from build123d import *

# Parameters (mm, degrees)
SKETCH1_R           = 63.5
BOSS_EXTRUDE1_DEPTH = 6.35
SKETCH2_R           = 20.6375
CUT_EXTRUDE1_DEPTH  = 91.02678768
SKETCH3_R           = 3.175
CUT_EXTRUDE2_DEPTH  = 91.02678768
SKETCH4_R           = 3.25
CUT_EXTRUDE3_DEPTH  = 91.02678768


with BuildPart() as part:
    # Sketch1 → Boss-Extrude1 (new body)
    with BuildSketch(Plane(origin=(0, 0, 0), x_dir=(1, 0, 0), z_dir=(0, 1, 0))):
        with Locations(Location((0, 0, 0), (0, 0, 270))):
            Circle(SKETCH1_R)
    extrude(amount=BOSS_EXTRUDE1_DEPTH)

    # Sketch2 → Cut-Extrude1 (cut, through all)
    with BuildSketch(Plane(origin=(0, 6.35, 0), x_dir=(1, 0, 0), z_dir=(0, 1, 0))):
        with Locations(Location((0, 0, 0), (0, 0, 270))):
            Circle(SKETCH2_R)
    extrude(amount=-CUT_EXTRUDE1_DEPTH, mode=Mode.SUBTRACT)

    # Sketch3 → Cut-Extrude2 (cut, through all)
    with BuildSketch(Plane(origin=(0, 6.35, 0), x_dir=(1, 0, 0), z_dir=(0, 1, 0))):
        with Locations(Location((-17.960512242, 17.960512242, 0), (0, 0, 270))):
            Circle(SKETCH3_R)
        with Locations(Location((17.960512242, 17.960512242, 0), (0, 0, 270))):
            Circle(SKETCH3_R)
        with Locations(Location((17.960512242, -17.960512242, 0), (0, 0, 270))):
            Circle(SKETCH3_R)
        with Locations(Location((-17.960512242, -17.960512242, 0), (0, 0, 270))):
            Circle(SKETCH3_R)
    extrude(amount=-CUT_EXTRUDE2_DEPTH, mode=Mode.SUBTRACT)

    # Sketch4 → Cut-Extrude3 (cut, through all)
    with BuildSketch(Plane(origin=(0, 6.35, 0), x_dir=(1, 0, 0), z_dir=(0, 1, 0))):
        with Locations(Location((-36.079282025, -1.812569594, 0), (0, 0, 270))):
            Circle(SKETCH4_R)
        with Locations(Location((2.429915675, 36.04296755, 0), (0, 0, 270))):
            Circle(SKETCH4_R)
        with Locations(Location((36.079282025, 1.812569594, 0), (0, 0, 270))):
            Circle(SKETCH4_R)
        with Locations(Location((-2.429915675, -36.04296755, 0), (0, 0, 270))):
            Circle(SKETCH4_R)
    extrude(amount=-CUT_EXTRUDE3_DEPTH, mode=Mode.SUBTRACT)


solid = part.part
Here's how the part is built. I have some questions about the finished solid (model axes, mm). Coordinates: 2 decimals unless noted, no trailing zeros. Order: outer loops, then holes, each group sorted by start corner. A loop starts at its lowest first (then second) coordinate and runs counter-clockwise, first axis right, second up. Notation, with made-up numbers: (-40, 72) -> (3, 72) arc R18 ccw to (3, 96) -> close; hole circle Ø11 at (38, 10). An arc over 180 degrees is marked (long way). Answer in a Markdown table with one row per item.
(1) I want a section at A-A on x = 4. List the corners of the cut face in (y, z) for me, then the cut area to 3 significant figures.
Answer key:
| item | result |
|---|---|
| outline | (0, -63.37) -> (6.35, -63.37) -> (6.35, -38.89) -> (0, -38.89) -> close; (0, -33.2) -> (6.35, -33.2) -> (6.35, -20.25) -> (0, -20.25) -> close; (0, 20.25) -> (6.35, 20.25) -> (6.35, 63.37) -> (0, 63.37) -> close |
| area | 512 mm^2 |
(2) I want a section at D-D on x = 55.5. List the corners of the cut face in (y, z) for me, then the cut area to 3 significant figures.
Answer key:
| item | result |
|---|---|
| outline | (0, -30.85) -> (6.35, -30.85) -> (6.35, 30.85) -> (0, 30.85) -> close |
| area | 392 mm^2 |
(3) Will these pins go through, and if not, where does the flat tip stop? pin 1 Ø5 at (x, z) = (-36.08, 1.81) entering from +Y; pin 2 Ø3 at (x, y) = (-28, 3.5) entering from -Z; pin 3 Ø2 at (y, z) = (2, -48.5) entering from -X.
Answer key:
| item | result |
|---|---|
| pin 1 | through |
| pin 2 | z = -57.71 |
| pin 3 | x = -42.14 |
(4) Thinking about a two-plate mould opening in X: for faces 1 (the face through (-61.99, 3.13, -13.77)), 2 (the face through (20.46, 3.22, -2.69)), 3 (the face through (15, 6.35, -15)), which applies, +X half, -X half, draft (parallel to the pull), parting line (faces both ways), or undercut?
Answer key:
| item | result |
|---|---|
| face 1 | parting line |
| face 2 | undercut |
| face 3 | draft |
(5) I want a section at C-C on y = 1.75. Count the separate pieces of the cut face and the enclosed holes in it, then the cut area to 3 significant figures.
Answer key:
| item | result |
|---|---|
| separate pieces | 1 |
| enclosed holes | 9 |
| area | 11,100 mm^2 |
(6) Please list where these lines run through material, in increasing order: probe 1 along X at (y, z) = (1, 4); probe 2 along X at (y, z) = (1.25, -1.5); probe 3 along X at (y, z) = (2.75, -17.5).
Answer key:
| item | result |
|---|---|
| probe 1 | -63.37 to -38.48, -33.68 to -20.25, 20.25 to 63.37 |
| probe 2 | -63.48 to -20.58, 20.58 to 32.84, 39.31 to 63.48 |
| probe 3 | -61.04 to -21.1, -14.82 to -10.94, 10.94 to 14.82, 21.1 to 61.04 |
(7) I want a section at B-B on z = 9. List the corners of the cut face in (x, y) for me, then the cut area to 3 significant figures.
Answer key:
| item | result |
|---|---|
| outline | (-62.86, 0) -> (-18.57, 0) -> (-18.57, 6.35) -> (-62.86, 6.35) -> close; (18.57, 0) -> (62.86, 0) -> (62.86, 6.35) -> (18.57, 6.35) -> close |
| area | 562 mm^2 |
